```python
from build123d import *

# Parameters (mm, degrees)
SKETCH1_W           = 500
SKETCH1_H           = 500
SKETCH1_R           = 1.525
SKETCH1_R_2         = 1.5
BOSS_EXTRUDE1_DEPTH = 6
BOSS_EXTRUDE2_DEPTH = 6
CUT_EXTRUDE1_DEPTH  = 7


with BuildPart() as part:
    # Sketch1 → Boss-Extrude1 (new body)
    with BuildSketch(Plane(origin=(0, 0, 0), x_dir=(1, 0, 0), z_dir=(0, 1, 0))):
        with Locations((250, -250)):
            Rectangle(SKETCH1_W, SKETCH1_H)
        with Locations((484, -20)):
            Circle(SKETCH1_R, mode=Mode.SUBTRACT)
        with Locations((16, -20)):
            Circle(SKETCH1_R_2, mode=Mode.SUBTRACT)
        with Locations((484, -469)):
            Circle(SKETCH1_R_2, mode=Mode.SUBTRACT)
        with Locations((16, -469)):
            Circle(SKETCH1_R_2, mode=Mode.SUBTRACT)
    extrude(amount=BOSS_EXTRUDE1_DEPTH)

    # Sketch2 → Boss-Extrude2 (add)
    with BuildSketch(Plane.XZ):
        Polygon((-6, 506), (-6, 0), (0, 0), (0, 500), (500, 500), (500, 0), (506, 0), (506, 506), align=None)
    extrude(amount=-BOSS_EXTRUDE2_DEPTH)

    # Sketch3 → Cut-Extrude1 (cut, through all)
    with BuildSketch(Plane.XZ):
        with BuildLine():
            Line((9, 60), (9, 260))
            ThreePointArc((9, 260), (14, 265), (19, 260))
            Line((19, 260), (19, 60))
            ThreePointArc((19, 60), (14, 55), (9, 60))
        make_face()
        with BuildLine():
            Line((491, 60), (491, 260))
            ThreePointArc((491, 260), (486, 265), (481, 260))
            Line((481, 260), (481, 60))
            ThreePointArc((481, 60), (486, 55), (491, 60))
        make_face()
    extrude(amount=-CUT_EXTRUDE1_DEPTH, mode=Mode.SUBTRACT)


solid = part.part
```
Geometry: final body of the model. Coordinates: model frame, mm. Round coordinates to 2 decimals unless told otherwise and drop trailing zeros. Write each loop counter-clockwise with the first axis right and the second up, starting at its lowest first coordinate (ties: lowest second). Pieces come first, ordered by that corner, then holes. Notation, with made-up numbers: M 86.5,38.5 L 119.5,38.5 A20 cw 119.5,59.5 Z; hole C 7,25.5 d8. An arc over 180 degrees is marked long. Answer in a Markdown table with one row per item. Add a question column.
(1) Cut plane B-B, the plane y = 2.75. Return the cut outline in (x, z) (3 decimals), then the cut area to 3 significant figures.
(2) Ray query, L1, parallel to X at y = 4.2, z = 469; L2, parallel to X at y = 4.25, z = 247.5; L3, parallel to Z at x = 484, y = 5.3 (3 decimals). Return the intervals inside material, ascending.
(3) Cut plane A-A, the plane z = 99.5. Return the cut outline in (x, y), then the cut area to 3 significant figures.
Established:
| question | item | result |
|---|---|---|
| 1 | outline | M -6,0 L 506,0 L 506,506 L -6,506 Z; hole M 9,60 A5 ccw 19,60 L 19,260 A5 ccw 9,260 Z; hole C 16,20 d3; hole C 16,469 d3; hole M 481,60 A5 ccw 491,60 L 491,260 A5 ccw 481,260 Z; hole C 484,20 d3.05; hole C 484,469 d3 |
| 1 | area | 255,000 mm² |
| 2 | L1 | -6 to 14.5, 17.5 to 482.5, 485.5 to 506 |
| 2 | L2 | -6 to 9, 19 to 481, 491 to 506 |
| 2 | L3 | 0 to 18.475, 21.525 to 55.417, 264.583 to 467.5, 470.5 to 506 |
| 3 | outline | M -6,0 L 9,0 L 9,6 L -6,6 Z; M 19,0 L 481,0 L 481,6 L 19,6 Z; M 491,0 L 506,0 L 506,6 L 491,6 Z |
| 3 | area | 2,950 mm² |
